Print and shaded views of the part. All mm, measured from the part's lowest x, y and z. A direction names the side the tool comes from. Round coordinates to 2 decimals unless told otherwise and drop trailing zeros. Loops run counter-clockwise (first coordinate to the right, second up) from the corner with the lowest first, then second, coordinate; pieces in that order, holes last. Notation, with made-up numbers: (19, 85.5) - (32, 85.5) arc R30 cw to (32, 123.5) - close; hole circle Ø4 at (63, 2.25). An arc over 180 degrees is marked (long way). Use one line per item in the form item = value.
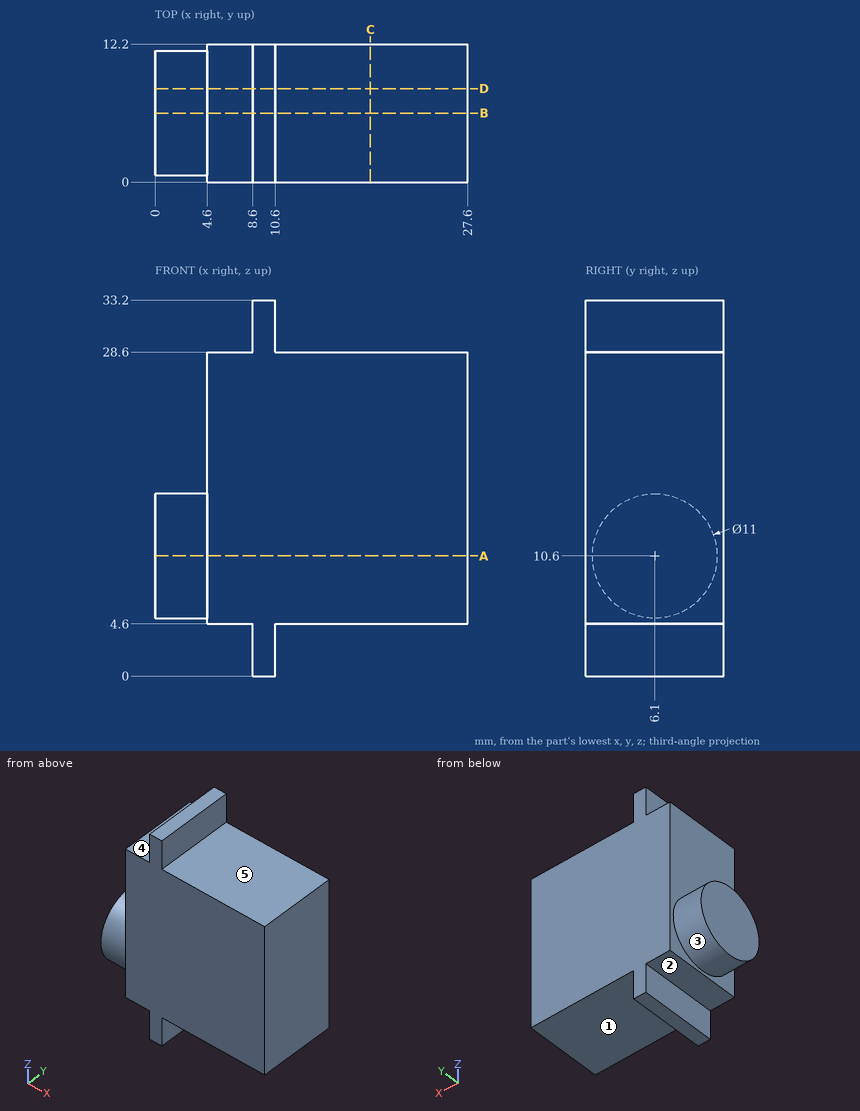
1. Cut at A-A, the plane z = 10.6. Give the cut face in (x, y), plus the area to 3 significant figures.
Geometry check:
outline = (0, 0.6) - (4.6, 0.6) - (4.6, 0) - (27.6, 0) - (27.6, 12.2) - (4.6, 12.2) - (4.6, 11.6) - (0, 11.6) - close
area = 331 mm^2
2. Tool access for the marked faces 1, 2, 3, 4 and 5: list every direction of +Z, -Z, +X, -X, +Y, -Y with a clear straight run to the whole face (end or side of a thin tool).
Geometry check:
face_1 = -Z, +X, +Y, -Y
face_2 = -Z, -X, +Y, -Y
face_3 = -X
face_4 = +Z, -X, +Y, -Y
face_5 = +Z, +X, +Y, -Y
3. Wall check: probe 1 along Z at (x, y) = (12, 5); probe 2 along X at (y, z) = (3, 24); probe 3 along Z at (x, y) = (4, 6). Give the ranges that are in metal, low to high.
Geometry check:
probe_1 = 4.6 to 28.6
probe_2 = 4.6 to 27.6
probe_3 = 5.1 to 16.1
4. Cut at D-D, the plane y = 8.25. Give the cut face in (x, z), plus the area to 3 significant figures.
Geometry check:
outline = (0, 5.54) - (4.6, 5.54) - (4.6, 4.6) - (8.6, 4.6) - (8.6, 0) - (10.6, 0) - (10.6, 4.6) - (27.6, 4.6) - (27.6, 28.6) - (10.6, 28.6) - (10.6, 33.2) - (8.6, 33.2) - (8.6, 28.6) - (4.6, 28.6) - (4.6, 15.66) - (0, 15.66) - close
area = 617 mm^2
5. Cut at C-C, the plane x = 19. Give the cut face in (y, z), plus the area to 3 significant figures.
Geometry check:
outline = (0, 4.6) - (12.2, 4.6) - (12.2, 28.6) - (0, 28.6) - close
area = 293 mm^2
6. Flat gauge pins, fed straight in: pin 1 (2 mm diameter, centred on x = 6.5, y = 3.5, fed in from +Z); pin 2 (5 mm diameter, centred on y = 5, z = 2.5, fed in from -X); pin 3 (1.4 mm diameter, centred on y = 8, z = 31.5, fed in from -X). Where does each tip first touch, or does it go through?
Geometry check:
pin_1 = 28.6
pin_2 = 4.6
pin_3 = 8.6
7. Cut at B-B, the plane y = 6.1. Give the cut face in (x, z), plus the area to 3 significant figures.
Geometry check:
outline = (0, 5.1) - (4.6, 5.1) - (4.6, 4.6) - (8.6, 4.6) - (8.6, 0) - (10.6, 0) - (10.6, 4.6) - (27.6, 4.6) - (27.6, 28.6) - (10.6, 28.6) - (10.6, 33.2) - (8.6, 33.2) - (8.6, 28.6) - (4.6, 28.6) - (4.6, 16.1) - (0, 16.1) - close
area = 621 mm^2
